Study the drawing (mm; zero at the part's minimum x, y, z) and answer. A direction names the side the tool comes from. Give positions to 0.01 mm unless a question says otherwise; leave off trailing zeros. Order: outer loops, then holes, each group sorted by start corner. A loop starts at its lowest first (then second) coordinate and runs counter-clockwise, first axis right, second up. Notation, with made-up numbers: (-19.5, 73.5) -> (10.5, 73.5) arc R34 ccw to (10.5, 112.5) -> close; hole circle Ø10 at (48.5, -10.75). An arc over 180 degrees is marked (long way). Answer as CSV lines item,"result". Start each with the question number.
1. A cutting plane is placed at D-D (x = 90). Give the vertices of the cut face in (y, z).
2. Find the intervals of material crossed by L1, parallel to Y at x = 52, z = 16; L2, parallel to Z at x = 44, y = 140; L3, parallel to Y at x = 117, z = 11.5, in increasing order.
3. A cutting plane is placed at C-C (z = 64). Give the vertices of the cut face in (x, y), then the cut area to 3 significant figures.
4. For the marked faces 5 and 6, determine the directions among +Z, -Z, +X, -X, +Y, -Y from which every point of the face is accessible in a straight line to the end or side of a thin tool.
5. A cutting plane is placed at B-B (x = 17). Give the vertices of the cut face in (y, z).
6. For a pull along Z with two mould halves and no side action, classify the marked faces 1, 2, 3 and 4 as released by +Z, released by -Z, zero draft, split by the parting line, or undercut.
7. A cutting plane is placed at A-A (y = 55.5). Give the vertices of the cut face in (x, z).
8. Flat-ended cylindrical pins translate along their axes: pin 1 (5 mm diameter, centred on y = 228.5, z = 38, fed in from +X); pin 2 (8 mm diameter, centred on x = 106, z = 122.5, fed in from +Y); pin 3 (2 mm diameter, centred on x = 76.5, z = 102, fed in from +Y). Find the tip coordinate at first contact, or state that the pin passes through.
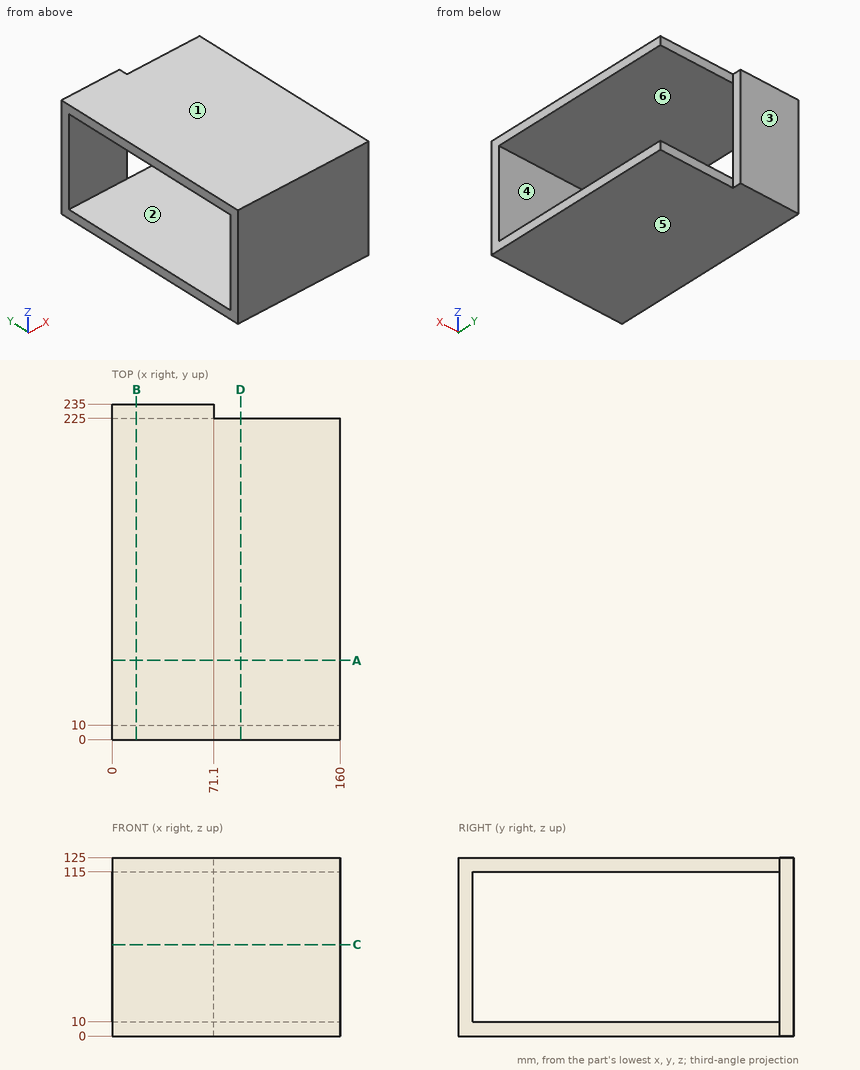
Answer sheet:
1,outline,"(0, 0) -> (225, 0) -> (225, 10) -> (10, 10) -> (10, 115) -> (225, 115) -> (225, 125) -> (0, 125) -> close"
2,L1,"y = 0 to 10, 225 to 235"
2,L2,"z = 0 to 10, 115 to 125"
2,L3,"y = 0 to 10"
3,outline,"(0, 0) -> (160, 0) -> (160, 10) -> (0, 10) -> close; (0, 225) -> (71.1, 225) -> (71.1, 235) -> (0, 235) -> close"
3,area,"2,310 mm^2"
4,face 5,"-Z, +X, -X, +Y, -Y"
4,face 6,"+X, -X"
5,outline,"(0, 0) -> (235, 0) -> (235, 125) -> (0, 125) -> close; hole (10, 10) -> (225, 10) -> (225, 115) -> (10, 115) -> close"
6,face 1,"released by +Z"
6,face 2,"undercut"
6,face 3,"zero draft"
6,face 4,"undercut"
7,outline,"(0, 0) -> (160, 0) -> (160, 10) -> (0, 10) -> close; (0, 115) -> (160, 115) -> (160, 125) -> (0, 125) -> close"
8,pin 1,"stops at x = 71.1"
8,pin 2,"stops at y = 225"
8,pin 3,"stops at y = 10"
